from build123d import *

# Parameters (mm, degrees)
BOSS_EXTRUDE1_DEPTH = 4
CUT_EXTRUDE1_START  = 6.5
CUT_EXTRUDE1_DEPTH  = 20.079745625
FILLET1_R           = 2
SKETCH2_R           = 0.8
SCREW_HOLES_DEPTH   = 13.579745788
SKETCH4_R           = 1.25
SCREW_HEADS_DEPTH   = 3


with BuildPart() as part:
    # Sketch5 → Boss-Extrude1 (new body)
    with BuildSketch(Plane(origin=(0, 0, 0), x_dir=(1, 0, 0), z_dir=(0, 1, 0))):
        with BuildLine():
            Line((-10, -6.5), (10, -6.5))
            Line((10, -6.5), (10, 4.202041029))
            ThreePointArc((10, 4.202041029), (0, 0), (-10, 4.202041029))
            Line((-10, 4.202041029), (-10, -6.5))
        make_face()
    extrude(amount=-BOSS_EXTRUDE1_DEPTH)

    # Sketch3 → Cut-Extrude1 (cut, through all)
    with BuildSketch(Plane.XY.offset(CUT_EXTRUDE1_START)):
        with BuildLine():
            Line((3, -4), (3, -2.5))
            ThreePointArc((3, -2.5), (2.560660172, -1.439339828), (1.5, -1))
            Line((1.5, -1), (-1.5, -1))
            ThreePointArc((-1.5, -1), (-2.560660172, -1.439339828), (-3, -2.5))
            Line((-3, -2.5), (-3, -4))
            Line((-3, -4), (0, -4))
            Line((0, -4), (3, -4))
        make_face()
    extrude(amount=-CUT_EXTRUDE1_DEPTH, mode=Mode.SUBTRACT)

    # Fillet1
    fillet1_edges = [part.edges().sort_by_distance(p)[0] for p in [
        (10, 0, 1.148979486),
        (-10, 0, 1.148979486),
    ]]
    fillet(fillet1_edges, radius=FILLET1_R)

    # Sketch2 → Screw Holes (cut, through all)
    with BuildSketch(Plane(origin=(0, 0, 0), x_dir=(1, 0, 0), z_dir=(0, 1, 0))):
        with Locations(Location((-8, -1.5, 0), (0, 0, 270))):
            Circle(SKETCH2_R)
        with Locations(Location((8, -1.5, 0), (0, 0, 270))):
            Circle(SKETCH2_R)
        with Locations(Location((8, -4.5, 0), (0, 0, 270))):
            Circle(SKETCH2_R)
        with Locations(Location((-8, -4.5, 0), (0, 0, 270))):
            Circle(SKETCH2_R)
    extrude(amount=-SCREW_HOLES_DEPTH, mode=Mode.SUBTRACT)

    # Sketch4 → Screw Heads (cut)
    with BuildSketch(Plane(origin=(0, 0, 0), x_dir=(1, 0, 0), z_dir=(0, 1, 0))):
        with Locations(Location((-8, -4.5, 0), (0, 0, 270))):
            Circle(SKETCH4_R)
        with Locations(Location((8, -4.5, 0), (0, 0, 270))):
            Circle(SKETCH4_R)
    extrude(amount=-SCREW_HEADS_DEPTH, mode=Mode.SUBTRACT)


solid = part.part
Build history of the part. All positions in model axes, mm. A direction names the side the tool comes from. Round coordinates to 2 decimals unless told otherwise and drop trailing zeros. Write each loop counter-clockwise with the first axis right and the second up, starting at its lowest first coordinate (ties: lowest second). Pieces come first, ordered by that corner, then holes. Notation, with made-up numbers: (89, 64.25) - (124, 64.25) arc R19 cw to (124, 93.25) - close; hole circle Ø1 at (-1.5, -18). An arc over 180 degrees is marked (long way). Use CSV: the item, a comma, the result in double quotes.
(1) Band-saw the part on C-C (x = 7.5). Write the cut outline in (y, z).
Response:
outline,"(-4, -2.18) - (0, -2.18) - (0, 0.88) - (-4, 0.88) - close; (-4, 2.12) - (0, 2.12) - (0, 3.35) - (-3, 3.35) - (-3, 3.88) - (-4, 3.88) - close; (-4, 5.12) - (-3, 5.12) - (-3, 5.65) - (0, 5.65) - (0, 6.5) - (-4, 6.5) - close"
(2) Mould opens along Z. For faces 4 (the cylindrical face through (8.793, -1.972, 1.396)), 5 (the flat face through (-10, -3, 1)), 6 (the cylindrical face through (0.2, -0.6, 0)) say: pulls with the +Z half, pulls with the -Z half, needs draft (parallel to the pull), parting line crosses it, or undercut.
Response:
face 4,"undercut"
face 5,"needs draft"
face 6,"pulls with the -Z half"
(3) Band-saw the part on B-B (z = 1.5). Write the cut outline in (x, y).
Response:
outline,"(-10, -4) - (-8.8, -4) - (-8.8, -0.17) arc R2 ccw to (-10, -2) - close; (-7.2, -4) - (-3, -4) - (-3, -2.5) arc R1.5 cw to (-1.5, -1) - (1.5, -1) arc R1.5 cw to (3, -2.5) - (3, -4) - (7.2, -4) - (7.2, 0) - (-7.2, 0) - close; (8.8, -4) - (10, -4) - (10, -2) arc R2 ccw to (8.8, -0.17) - close"
(4) Wall check: line 1 (X direction, y = -2.95, z = 1.5); line 2 (X direction, y = -2.3, z = 4); line 3 (Y direction, x = 0.5, z = 2). Give the ranges that are in metal, low to high.
Response:
line 1,"-10 to -8.8, -7.2 to -3, 3 to 7.2, 8.8 to 10"
line 2,"-10 to -9.15, -6.85 to -2.99, 2.99 to 6.85, 9.15 to 10"
line 3,"-1 to 0"
(5) Band-saw the part on D-D (y = -0.6). Write the cut outline in (x, z).
Response:
outline,"(-9.43, -3.65) arc R14 cw to (9.43, -3.65) - (9.43, 6.5) - (-9.43, 6.5) - close; hole circle Ø2.5 at (-8, 4.5); hole circle Ø1.6 at (-8, 1.5); hole circle Ø2.5 at (8, 4.5); hole circle Ø1.6 at (8, 1.5)"
(6) Pin check, flat tips, straight feed: P1, Ø1, axis at x = -8, z = 1.5, coming from the -Y side; P2, Ø2.5, axis at x = -0.5, z = 4.5, coming from the -Y side; P3, Ø2, axis at x = -8, z = 4.5, coming from the +Y side. Stop position of each tip, or through.
Response:
P1,"through"
P2,"y = -1.02"
P3,"y = -3"
(7) Band-saw the part on A-A (y = -3.35). Write the cut outline in (x, z).
Response:
outline,"(-10, -4.2) arc R14 cw to (-3, -0.33) - (-3, 6.5) - (-10, 6.5) - close; (3, -0.33) arc R14 cw to (10, -4.2) - (10, 6.5) - (3, 6.5) - close; hole circle Ø1.6 at (-8, 1.5); hole circle Ø1.6 at (-8, 4.5); hole circle Ø1.6 at (8, 1.5); hole circle Ø1.6 at (8, 4.5)"
(8) 3-axis set-ups, long thin cutter, end or side, ignore diameter. For faces 1 (the flat face through (0, -1, 3)), 2 (the cylindrical face through (9.6, -0.8, 1.1)), 3 (the cylindrical face through (6.78, -1.48, 4.23)): which of +Z, -Z, +X, -X, +Y, -Y reach the whole face in a straight line?
Response:
face 1,"+Z, -Z, -Y"
face 2,"+Z, -Z, +X, +Y"
face 3,"+Y"
